Build history of the part. All positions in model axes, mm. A direction names the side the tool comes from. Round coordinates to 2 decimals unless told otherwise and drop trailing zeros. Order: outer loops, then holes, each group sorted by start corner. A loop starts at its lowest first (then second) coordinate and runs counter-clockwise, first axis right, second up. Notation, with made-up numbers: M 40,-4.75 L 57,-4.75 A24 ccw 57,33.25 Z; hole C -16,-39.75 d4. An arc over 180 degrees is marked long. One line per item, written item: value. Start each with the question number.
Item 1: Two-plate mould, pull along Y, no slides. Class faces 1 (the flat face through (1.4, -1.4, 4)), 2 (the flat face through (-1.5, 0, 2)), 3 (the cylindrical face through (0, 2, -2)): +Y half, -Y half, draft (parallel to the pull), parting line (faces both ways), or undercut.
Item 2: Pin check, flat tips, straight feed: pin 1 (1.5 mm diameter, centred on y = 2, z = 1, fed in from -X); pin 2 (1.5 mm diameter, centred on y = -1, z = -0.5, fed in from +X); pin 3 (1 mm diameter, centred on x = 3, z = -2.5, fed in from -Y); pin 4 (0.5 mm diameter, centred on y = 0.5, z = 2, fed in from -X). Stop position of each tip, or through.
Item 3: Tool access for faces 4 (the cylindrical face through (3.233, -1.341, 1.976)), 5 (the flat face through (0.76, 1.293, 2.394)), 6 (the flat face through (1, -2, 0)): list every direction of +Z, -Z, +X, -X, +Y, -Y with a clear straight run to the whole face (end or side of a thin tool).
Item 4: Band-saw the part on B-B, the plane y = 0. Write the cut outline in (x, z).
Item 5: Band-saw the part on A-A, the plane z = 3.5. Write the cut outline in (x, y).
Item 6: Probe L1, parallel to X at y = -1, z = -4; L2, parallel to Z at x = 0.25, y = 3.25; L3, parallel to Y at x = 0.25, z = 3. List the from-to ranges inside material, lowest first.
Item 7: Band-saw the part on C-C, the plane z = -1.25. Write the cut outline in (x, y).
```python
from build123d import *

# Parameters (mm, degrees)
F0_R     = 3.5
F1_DEPTH = 4
F2_R     = 2
F3_DEPTH = 5
F5_DEPTH = 3
F6_R     = 0.25


with BuildPart() as f1:
    # F0 (on Top) → F1 (new body)
    with BuildSketch(Plane.XY):
        Circle(F0_R)
    extrude(amount=F1_DEPTH)

    # F2 (on face) → F3 (join)
    with BuildSketch(Plane(origin=(0, 0, 0), x_dir=(1, 0, 0), z_dir=(0, 0, -1))):
        Circle(F2_R)
    extrude(amount=F3_DEPTH)

    # F4 (on face) → F5 (cut)
    with BuildSketch(Plane.XY.offset(4)):
        Polygon((1.5, -0.8660254038), (1.5, 0.8660254038), (0, 1.7320508076), (-1.5, 0.8660254038), (-1.5, -0.8660254038), (0, -1.7320508076), align=None)
    extrude(amount=-F5_DEPTH, mode=Mode.SUBTRACT)

    # F6
    f6_edges = [f1.edges().sort_by_distance(p)[0] for p in [
        (-3.5, 0, 4),
        (1.5, 0, 4),
        (0.75, 1.299038, 4),
        (-0.75, 1.299038, 4),
        (-1.5, 0, 4),
        (-0.75, -1.299038, 4),
        (0.75, -1.299038, 4),
        (-3.5, 0, 0),
    ]]
    fillet(f6_edges, radius=F6_R)


solid = f1.part
```
Output:
1. face 1: draft
1. face 2: undercut
1. face 3: parting line
2. pin 1: stops at x = -3.27
2. pin 2: stops at x = 3.42
2. pin 3: passes through
2. pin 4: stops at x = -3.49
3. face 4: +Z, -Z
3. face 5: +Z
3. face 6: -Z
4. outline: M -3.5,0.25 A0.25 ccw -3.25,0 L -2,0 L -2,-5 L 2,-5 L 2,0 L 3.25,0 A0.25 ccw 3.5,0.25 L 3.5,3.75 A0.25 ccw 3.25,4 L 1.75,4 A0.25 ccw 1.5,3.75 L 1.5,1 L -1.5,1 L -1.5,3.75 A0.25 ccw -1.75,4 L -3.25,4 A0.25 ccw -3.5,3.75 Z
5. outline: C 0,0 d7; hole M -1.5,-0.87 L 0,-1.73 L 1.5,-0.87 L 1.5,0.87 L 0,1.73 L -1.5,0.87 Z
6. L1: x = -1.73 to 1.73
6. L2: z = 0 to 4
6. L3: y = -3.49 to -1.59, 1.59 to 3.49
7. outline: C 0,0 d4
